The figure shows three views and two pictorial views of one solid part (mm, origin at its lowest corner). Answer the questions. A direction names the side the tool comes from. Round coordinates to 2 decimals unless told otherwise and drop trailing zeros. Order: outer loops, then holes, each group sorted by start corner. A loop starts at its lowest first (then second) coordinate and runs counter-clockwise, first axis right, second up. Notation, with made-up numbers: (14, 86.5) - (42, 86.5) arc R22 ccw to (42, 94.5) - close; hole circle Ø5 at (-19.5, 67.5). An arc over 180 degrees is marked (long way). Use CSV: the item, a comma, the result in double quotes.
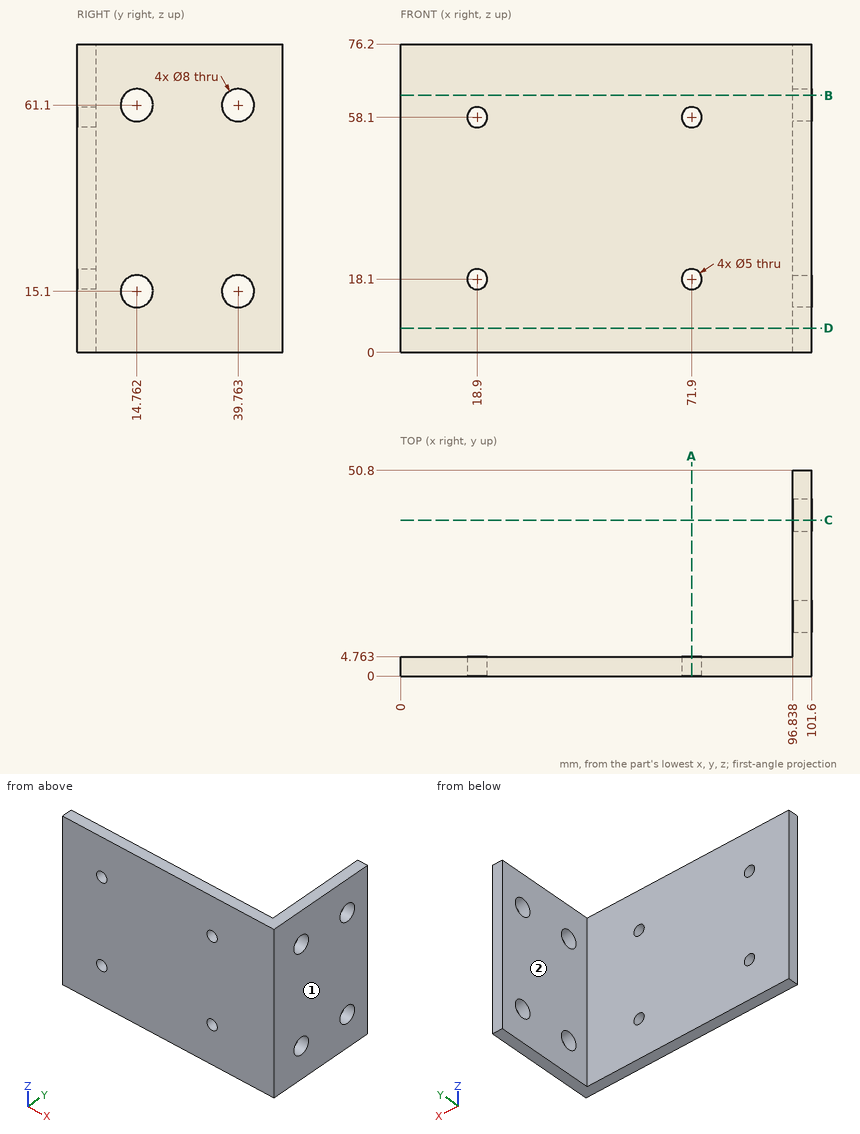
(1) Find section A-A (x = 71.9). Determine the outline of the cut face in (y, z).
Findings below:
outline,"(0, 0) - (4.76, 0) - (4.76, 15.6) - (0, 15.6) - close; (0, 20.6) - (4.76, 20.6) - (4.76, 55.6) - (0, 55.6) - close; (0, 60.6) - (4.76, 60.6) - (4.76, 76.2) - (0, 76.2) - close"
(2) Find section C-C (y = 38.5). Determine the outline of the cut face in (x, z) (1 decimal).
Findings below:
outline,"(96.8, 0) - (101.6, 0) - (101.6, 11.3) - (96.8, 11.3) - close; (96.8, 18.9) - (101.6, 18.9) - (101.6, 57.3) - (96.8, 57.3) - close; (96.8, 64.9) - (101.6, 64.9) - (101.6, 76.2) - (96.8, 76.2) - close"
(3) For the marked faces 1 and 2, determine the directions among +Z, -Z, +X, -X, +Y, -Y from which every point of the face is accessible in a straight line to the end or side of a thin tool.
Findings below:
face 1,"+Z, -Z, +X, +Y, -Y"
face 2,"+Z, -Z, -X, +Y"
(4) Find section B-B (z = 63.5). Determine the outline of the cut face in (x, y).
Findings below:
outline,"(0, 0) - (101.6, 0) - (101.6, 11.56) - (96.84, 11.56) - (96.84, 4.76) - (0, 4.76) - close; (96.84, 17.96) - (101.6, 17.96) - (101.6, 36.56) - (96.84, 36.56) - close; (96.84, 42.96) - (101.6, 42.96) - (101.6, 50.8) - (96.84, 50.8) - close"
(5) Find section D-D (z = 6). Determine the outline of the cut face in (x, y), and give its area (3 significant figures).
Findings below:
outline,"(0, 0) - (101.6, 0) - (101.6, 50.8) - (96.84, 50.8) - (96.84, 4.76) - (0, 4.76) - close"
area,"703 mm²"
(6) Each of these flat-tipped pins is pushed along its axis until it touches: pin 1 (4 mm diameter, centred on x = 18.9, z = 18.1, fed in from -Y); pin 2 (6 mm diameter, centred on x = 18.9, z = 58.1, fed in from -Y); pin 3 (10 mm diameter, centred on y = 26.5, z = 67.5, fed in from -X). Where does it stop, or does it pass through?
Findings below:
pin 1,"passes through"
pin 2,"stops at y = 0"
pin 3,"stops at x = 96.84"
(7) Find the intervals of material crossed by L1, parallel to Y at x = 99, z = 15; L2, parallel to Z at x = 18.9, y = 1.3; L3, parallel to X at y = 1, z = 58, in increasing order. Write a range as from..to.
Findings below:
L1,"y = 0..10.76, 18.76..35.76, 43.76..50.8"
L2,"z = 0..15.6, 20.6..55.6, 60.6..76.2"
L3,"x = 0..16.4, 21.4..69.4, 74.4..101.6"
